from build123d import *

# Parameters (mm, degrees)
F0_W     = 7.8
F0_H     = 5
F0_W_2   = 4.4
F1_DEPTH = 3
F2_DEPTH = 12
F3_DEPTH = 8
F4_SIZE  = 2
F5_SIZE  = 4.5
F6_SIZE  = 3
F7_SIZE  = 1


with BuildPart() as f1:
    # F0 (on Top) → F1 (new body)
    with BuildSketch(Plane.XY):
        Polygon((0, 15), (0, 10), (7.8, 10), (12.2, 10), (20, 10), (20, 15), align=None)
        with Locations((3.9, 7.5)):
            Rectangle(F0_W, F0_H)
        with Locations((10, 7.5)):
            Rectangle(F0_W_2, F0_H)
        with Locations((16.1, 7.5)):
            Rectangle(F0_W, F0_H)
        Polygon((0, 5), (0, 0), (20, 0), (20, 5), (12.2, 5), (7.8, 5), align=None)
    extrude(amount=-F1_DEPTH)

    # F0 (on Top) → F2 (join)
    with BuildSketch(Plane.XY):
        with Locations((3.9, 7.5)):
            Rectangle(F0_W, F0_H)
        with Locations((16.1, 7.5)):
            Rectangle(F0_W, F0_H)
    extrude(amount=F2_DEPTH)

    # F0 (on Top) → F3 (join)
    with BuildSketch(Plane.XY):
        with Locations((10, 7.5)):
            Rectangle(F0_W_2, F0_H)
    extrude(amount=F3_DEPTH)

    # F4
    f4_edges = [f1.edges().sort_by_distance(p)[0] for p in [
        (0, 10, 6),
        (0, 5, 6),
        (20, 5, 6),
        (20, 10, 6),
    ]]
    chamfer(f4_edges, length=F4_SIZE)

    # F5
    f5_edges = [f1.edges().sort_by_distance(p)[0] for p in [
        (0, 7.5, 12),
        (20, 7.5, 12),
    ]]
    chamfer(f5_edges, length=F5_SIZE)

    # F6
    f6_edges = [f1.edges().sort_by_distance(p)[0] for p in [
        (0, 15, -1.5),
        (0, 0, -1.5),
        (20, 0, -1.5),
        (20, 15, -1.5),
    ]]
    chamfer(f6_edges, length=F6_SIZE)

    # F7
    f7_edges = [f1.edges().sort_by_distance(p)[0] for p in [
        (10, 5, 8),
        (10, 10, 8),
    ]]
    chamfer(f7_edges, length=F7_SIZE)


solid = f1.part
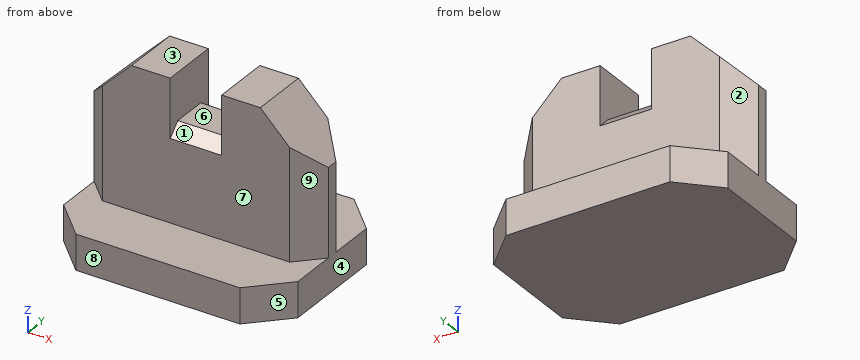
Geometry check sheet. Reference: the model listing, model coordinates, mm. Face numbers are marked on the shaded views. A direction names the side the tool comes from. Coordinates: 2 decimals unless noted, no trailing zeros. Order: outer loops, then holes, each group sorted by start corner. A loop starts at its lowest first (then second) coordinate and runs counter-clockwise, first axis right, second up. Notation, with made-up numbers: (41.5, 4) - (65.5, 4) arc R16 cw to (65.5, 23) - close; hole circle Ø11 at (62, 47). An arc over 180 degrees is marked (long way). Answer in a Markdown table with one row per item. Add a question column.
1) Cross-section at C-C, the plane x = 7.5. Record the cut outline in (y, z), then the cut area to 3 significant figures.
2) Gauge pin test, flat ends, axial feed: P1, Ø2, axis at x = 12.5, z = 8.5, coming from the -Y side; P2, Ø4, axis at y = 6.5, z = 9.5, coming from the -X side; P3, Ø6, axis at x = 7, z = 8.5, coming from the +Y side; P4, Ø1.5, axis at y = 12.5, z = 0.5, coming from the -X side. Record the tip position at first contact, or that the pin passes through.
3) Cross-section at D-D, the plane z = 4.5. Record the cut outline in (x, y).
4) Cross-section at A-A, the plane z = 10. Record the cut outline in (x, y).
5) Set-up check for the marked faces 5, 6, 7, 8 and 9: record each of +Z, -Z, +X, -X, +Y, -Y from which the full face is reachable in a straight line by a thin tool's end or side.
6) Material ranges on line 1 along Z through (x, y) = (5.75, 4.25); line 2 along Y through (x, z) = (10, 4.25); line 3 along Z through (x, y) = (18, 8.75), recorded low to high. Write a range as [from, to].
7) Release check for a two-part mould opening along X. For the marked faces 1, 2, 3 and 4 record: +X half, -X half, draft (parallel to the pull), parting line (faces both ways), or undercut.
8) Cross-section at B-B, the plane y = 6.5. Record the cut outline in (x, z).
Check result:
| question | item | result |
|---|---|---|
| 1 | outline | (0, -3) - (15, -3) - (15, 0) - (10, 0) - (10, 12) - (5, 12) - (5, 0) - (0, 0) - close |
| 1 | area | 105 mm² |
| 2 | P1 | stops at y = 5 |
| 2 | P2 | stops at x = 0.05 |
| 2 | P3 | stops at y = 10 |
| 2 | P4 | stops at x = 0 |
| 3 | outline | (0, 7) - (2, 5) - (18, 5) - (20, 7) - (20, 8) - (18, 10) - (2, 10) - (0, 8) - close |
| 4 | outline | (2.5, 5) - (7.8, 5) - (7.8, 10) - (2.5, 10) - close; (12.2, 5) - (17.5, 5) - (17.5, 10) - (12.2, 10) - close |
| 5 | face 5 | +Z, -Z, +X, -Y |
| 5 | face 6 | +Z, +Y, -Y |
| 5 | face 7 | +Z, +X, -X, -Y |
| 5 | face 8 | +Z, -Z, +X, -X, -Y |
| 5 | face 9 | +Z, +X, -Y |
| 6 | line 1 | z = [-3, 0] |
| 6 | line 2 | y = [5, 10] |
| 6 | line 3 | z = [-3, 9.5] |
| 7 | face 1 | undercut |
| 7 | face 2 | -X half |
| 7 | face 3 | draft |
| 7 | face 4 | +X half |
| 8 | outline | (0, -3) - (20, -3) - (20, 0) - (19.5, 0) - (19.5, 8) - (15.5, 12) - (12.2, 12) - (12.2, 8) - (7.8, 8) - (7.8, 12) - (4.5, 12) - (0.5, 8) - (0.5, 0) - (0, 0) - close |
